Part model, mm, in its own coordinate system. A direction names the side the tool comes from. Round coordinates to 2 decimals unless told otherwise and drop trailing zeros. Write each loop counter-clockwise with the first axis right and the second up, starting at its lowest first coordinate (ties: lowest second). Pieces come first, ordered by that corner, then holes. Notation, with made-up numbers: M -27,55.5 L 15,55.5 A28 cw 15,92.5 Z; hole C 65.5,64 d8. An arc over 180 degrees is marked long. One line per question, with ' | ' between items. Start each with the question number.
1) Saw through at B-B (x = -8.5). List the corners of the cut face in (y, z).
2) Tool access for faces 4 (the face through (0, 213, 7)), 5 (the face through (-0.64, -52.12, 1.48)): list every direction of +Z, -Z, +X, -X, +Y, -Y with a clear straight run to the whole face (end or side of a thin tool).
3) Saw through at C-C (z = 1.75). Give the number of separate pieces and of enclosed holes in the cut face, plus the area to 3 significant figures.
4) Wall check: probe 1 along Y at (x, z) = (0, 1.95); probe 2 along Y at (x, z) = (20.5, 3.25); probe 3 along Y at (x, z) = (4, 0.5). Give the ranges that are in metal, low to high. Write a range as [from, to].
5) Saw through at A-A (y = 0). List the corners of the cut face in (x, z).
6) Drop flat-ended pins along their axis: pin 1 Ø0.6 at (y, z) = (213, 6.5) entering from -X; pin 2 Ø4 at (x, y) = (28.5, 86.5) entering from +Z; pin 3 Ø0.6 at (y, z) = (212.5, 6) entering from +X. Give the stop position or say it passes through.
7) Mould opens along Y. For faces 1 (the face through (-32.473, 79.35, 2.465)), 2 (the face through (2, 215, 3)), 3 (the face through (0, -52, 7)) say: pulls with the +Y half, pulls with the -Y half, needs draft (parallel to the pull), parting line crosses it, or undercut.
8) Saw through at D-D (y = -29.5). List the corners of the cut face in (x, z), plus the area to 3 significant figures.
```python
from build123d import *

# Parameters (mm, degrees)
SKETCH_R        = 32
PAD_DEPTH       = 5
PAD001_DEPTH    = 2
SKETCH002_R     = 1.7
POCKET_DEPTH    = 7.001
SKETCH003_R     = 2.95
POCKET001_DEPTH = 3
SKETCH004_R     = 1.7
POCKET002_DEPTH = 7.001


with BuildPart() as part:
    # Sketch → Pad (new body)
    with BuildSketch(Plane.XY):
        with BuildLine():
            ThreePointArc((-47.293619, 36.923077), (0, -60), (47.293619, 36.923077))
            ThreePointArc((47.293619, 123.076923), (32.469508, 80), (47.293619, 36.923077))
            ThreePointArc((47.293619, 123.076923), (3.1e-05, 220), (-47.293657, 123.076972))
            ThreePointArc((-47.293619, 36.923077), (-32.469508, 80.000031), (-47.293657, 123.076972))
        make_face()
        Circle(SKETCH_R, mode=Mode.SUBTRACT)
        with Locations((0, 160)):
            Circle(SKETCH_R, mode=Mode.SUBTRACT)
    extrude(amount=PAD_DEPTH)

    # Sketch001 (on Face8 of Pad) → Pad001 (join)
    with BuildSketch(Plane.XY.offset(5)):
        with BuildLine():
            Line((-5, -59.791304), (-5, -45))
            Line((-5, -45), (5, -45))
            Line((5, -45), (5, -59.791304))
            ThreePointArc((-5, -59.791304), (0, -60), (5, -59.791304))
        make_face()
        with BuildLine():
            ThreePointArc((5, 219.791304), (0, 220), (-5, 219.791304))
            Line((-5, 219.791304), (-5, 205))
            Line((-5, 205), (5, 205))
            Line((5, 205), (5, 219.791304))
        make_face()
    extrude(amount=PAD001_DEPTH)

    # Sketch002 (on Face14 of Pad001) → Pocket (cut, through all)
    with BuildSketch(Plane.XY.offset(7)):
        with Locations((0, -55)):
            Circle(SKETCH002_R)
        with Locations((0, 215)):
            Circle(SKETCH002_R)
    extrude(amount=-POCKET_DEPTH, mode=Mode.SUBTRACT)

    # Sketch003 (on Face4 of Pocket) → Pocket001 (cut)
    with BuildSketch(Plane(origin=(0, 0, 0), x_dir=(1, 0, 0), z_dir=(0, 0, -1))):
        with Locations((0, 55)):
            Circle(SKETCH003_R)
        with Locations((0, -215)):
            Circle(SKETCH003_R)
    extrude(amount=-POCKET001_DEPTH, mode=Mode.SUBTRACT)

    # Sketch004 (on Face4 of Pocket001) → Pocket002 (cut, through all)
    with BuildSketch(Plane(origin=(0, 0, 0), x_dir=(1, 0, 0), z_dir=(0, 0, -1))):
        with Locations((28.5, -73.5)):
            Circle(SKETCH004_R)
        with Locations((28.5, -86.5)):
            Circle(SKETCH004_R)
        with Locations((-28.5, -86.5)):
            Circle(SKETCH004_R)
        with Locations((-28.5, -73.5)):
            Circle(SKETCH004_R)
    extrude(amount=-POCKET002_DEPTH, mode=Mode.SUBTRACT)


solid = part.part
```
Answer key:
1) outline: M -59.39,0 L -30.85,0 L -30.85,5 L -59.39,5 Z; M 30.85,0 L 129.15,0 L 129.15,5 L 30.85,5 Z; M 190.85,0 L 219.39,0 L 219.39,5 L 190.85,5 Z
2) face 4: +Z, +X, -X, +Y, -Y | face 5: -Z
3) separate pieces: 1 | enclosed holes: 8 | area: 19,500 mm2
4) probe 1: y = [-60, -57.95], [-52.05, -32], [32, 128], [192, 212.05], [217.95, 220] | probe 2: y = [-56.39, -24.57], [24.57, 135.43], [184.57, 216.39] | probe 3: y = [-59.87, -31.75], [31.75, 128.25], [191.75, 219.87]
5) outline: M -60,0 L -32,0 L -32,5 L -60,5 Z; M 32,0 L 60,0 L 60,5 L 32,5 Z
6) pin 1: stops at x = -5 | pin 2: stops at z = 5 | pin 3: stops at x = 5
7) face 1: undercut | face 2: undercut | face 3: needs draft
8) outline: M -52.25,0 L -12.4,0 L -12.4,5 L -52.25,5 Z; M 12.4,0 L 52.25,0 L 52.25,5 L 12.4,5 Z | area: 398 mm2
